Work out the finished part from the listing and answer in its coordinate system (mm). Face numbers are marked on the shaded views. A direction names the side the tool comes from. Coordinates: 2 decimals unless noted, no trailing zeros. Order: outer loops, then holes, each group sorted by start corner. A loop starts at its lowest first (then second) coordinate and runs counter-clockwise, first axis right, second up. Notation, with made-up numbers: (40, -37.5) - (90, -37.5) arc R22 cw to (90, -0.5) - close; hole circle Ø2 at (62.25, 45). An arc over 180 degrees is marked (long way). Answer as a JSON object with one key per item and string values. Group by question number.
1) Section D-D (x = -2.5) is taken. Give the vertices of the cut face in (y, z), plus the area to 3 significant figures.
2) A tool of negligible diameter and unlimited length cuts with its end or side. For the marked faces 5, 6, 7, 8 and 9, from which of +Z, -Z, +X, -X, +Y, -Y can it reach the whole face along a straight path? Write none if from no direction.
3) Each of these flat-tipped pins is pushed along its axis until it touches: P1, Ø1.6, axis at x = 3, y = 0, coming from the -Z side; P2, Ø1, axis at x = -4.5, y = 2, coming from the -Z side; P3, Ø0.9, axis at y = 1, z = 13, coming from the +X side. Where does it stop, or does it pass through?
4) Section B-B (y = -3) is taken. Give the vertices of the cut face in (x, z).
5) The mould has two halves that part along X. Classify the marked faces 1, 2, 3 and 4: released by +X, released by -X, zero draft, split by the parting line, or undercut.
6) Find the intervals of material crossed by line 1 along Y through (x, z) = (8, 11.65); line 2 along Y through (x, z) = (0, 14.5); line 3 along X through (y, z) = (2, 1), in increasing order.
7) Section A-A (x = 8) is taken. Give the vertices of the cut face in (y, z), plus the area to 3 significant figures.
8) Section C-C (z = 9.5) is taken. Give the vertices of the cut face in (x, y), plus the area to 3 significant figures.
from build123d import *

# Parameters (mm, degrees)
PAD_DEPTH       = 15
SKETCH001_W     = 18
SKETCH001_H     = 8
POCKET_DEPTH    = 14
SKETCH002_R     = 1
PAD001_DEPTH    = 2
SKETCH003_R     = 0.5
POCKET001_DEPTH = 15.001
SKETCH004_W     = 8
SKETCH004_H     = 5
SKETCH004_R     = 1.25
PAD002_DEPTH    = 4
SKETCH005_W     = 3.5
SKETCH005_H     = 3
POCKET002_DEPTH = 2.5
POCKET003_DEPTH = 7.501
SKETCH007_W     = 3.5
SKETCH007_H     = 8
PAD003_DEPTH    = 3
SKETCH008_W     = 3
SKETCH008_H     = 3
POCKET004_DEPTH = 2.5
SKETCH010_R     = 0.5
POCKET005_DEPTH = 12.501
SKETCH011_R     = 0.5
POCKET006_DEPTH = 15.001
SKETCH012_W     = 1.058742
SKETCH012_H     = 1
SKETCH012_W_2   = 1.116308
POCKET007_DEPTH = 1


with BuildPart() as part:
    # Sketch → Pad (new body)
    with BuildSketch(Plane.XY):
        with BuildLine():
            Line((-10, 5), (10, 5))
            Line((10, 5), (10, 1.5))
            ThreePointArc((10, -1.5), (11.5, 0), (10, 1.5))
            Line((10, -1.5), (10, -5))
            Line((10, -5), (-10, -5))
            Line((-10, -5), (-10, -1.5))
            ThreePointArc((-10, 1.5), (-11.5, 0), (-10, -1.5))
            Line((-10, 1.5), (-10, 5))
        make_face()
    extrude(amount=PAD_DEPTH)

    # Sketch001 (on Face9 of Pad) → Pocket (cut)
    with BuildSketch(Plane(origin=(0, 0, 0), x_dir=(1, 0, 0), z_dir=(0, 0, -1))):
        Rectangle(SKETCH001_W, SKETCH001_H)
    extrude(amount=-POCKET_DEPTH, mode=Mode.SUBTRACT)

    # Sketch002 (on Face15 of Pocket) → Pad001 (join)
    with BuildSketch(Plane(origin=(0, 0, 14), x_dir=(1, 0, 0), z_dir=(0, 0, -1))):
        with Locations((-2.5, 0)):
            Circle(SKETCH002_R)
        with Locations((2.5, 0)):
            Circle(SKETCH002_R)
    extrude(amount=PAD001_DEPTH)

    # Sketch003 (on Face5 of Pad001) → Pocket001 (cut, through all)
    with BuildSketch(Plane.XY.offset(15)):
        Circle(SKETCH003_R)
    extrude(amount=-POCKET001_DEPTH, mode=Mode.SUBTRACT)

    # Sketch004 (on Face5 of Pocket001) → Pad002 (join)
    with BuildSketch(Plane.XY.offset(15)):
        Rectangle(SKETCH004_W, SKETCH004_H)
        Circle(SKETCH004_R, mode=Mode.SUBTRACT)
    extrude(amount=PAD002_DEPTH)

    # Sketch005 (on Face20 of Pad002) → Pocket002 (cut)
    with BuildSketch(Plane.XY.offset(19)):
        Rectangle(SKETCH005_W, SKETCH005_H)
    extrude(amount=-POCKET002_DEPTH, mode=Mode.SUBTRACT)

    # Sketch006 (on Face16 of Pocket002) → Pocket003 (cut, through all)
    with BuildSketch(Plane.XZ.offset(2.5)):
        with BuildLine():
            ThreePointArc((0.15, 19.022961), (0, 19.172961), (-0.15, 19.022961))
            Line((-0.15, 19.022961), (-0.15, 16.673611))
            ThreePointArc((-0.15, 16.673611), (0, 16.523611), (0.15, 16.673611))
            Line((0.15, 16.673611), (0.15, 19.022961))
        make_face()
    extrude(amount=-POCKET003_DEPTH, mode=Mode.SUBTRACT)

    # Sketch007 (on Face19 of Pocket003) → Pad003 (join)
    with BuildSketch(Plane(origin=(0, 0, 14), x_dir=(1, 0, 0), z_dir=(0, 0, -1))):
        with Locations((7.25, 0)):
            Rectangle(SKETCH007_W, SKETCH007_H)
        with Locations((-7.25, 0)):
            Rectangle(SKETCH007_W, SKETCH007_H)
    extrude(amount=PAD003_DEPTH)

    # Sketch008 (on Face5 of Pad003) → Pocket004 (cut)
    with BuildSketch(Plane.XY.offset(15)):
        with Locations((8.5, -3.5)):
            Rectangle(SKETCH008_W, SKETCH008_H)
        with Locations((8.5, 3.5)):
            Rectangle(SKETCH008_W, SKETCH008_H)
        with Locations((-8.5, -3.5)):
            Rectangle(SKETCH008_W, SKETCH008_H)
        with Locations((-8.5, 3.5)):
            Rectangle(SKETCH008_W, SKETCH008_H)
    extrude(amount=-POCKET004_DEPTH, mode=Mode.SUBTRACT)

    # Sketch010 → Pocket005 (cut, through all)
    with BuildSketch(Plane.XY.offset(12.5)):
        with Locations((8, -3)):
            Circle(SKETCH010_R)
        with Locations((8, 3)):
            Circle(SKETCH010_R)
        with Locations((-8, 3)):
            Circle(SKETCH010_R)
        with Locations((-8, -3)):
            Circle(SKETCH010_R)
    extrude(amount=-POCKET005_DEPTH, mode=Mode.SUBTRACT)

    # Sketch011 (on Face6 of Pocket005) → Pocket006 (cut, through all)
    with BuildSketch(Plane.XY.offset(15)):
        with Locations((-10, 0)):
            Circle(SKETCH011_R)
        with Locations((10, 0)):
            Circle(SKETCH011_R)
    extrude(amount=-POCKET006_DEPTH, mode=Mode.SUBTRACT)

    # Sketch012 (on Face2 of Pocket006) → Pocket007 (cut)
    with BuildSketch(Plane(origin=(0, 0, 0), x_dir=(1, 0, 0), z_dir=(0, 0, -1))):
        with Locations((-9.46722, -1.2e-05)):
            Rectangle(SKETCH012_W, SKETCH012_H)
        with Locations((9.416079, -0.000664)):
            Rectangle(SKETCH012_W_2, SKETCH012_H)
    extrude(amount=-POCKET007_DEPTH, mode=Mode.SUBTRACT)


solid = part.part
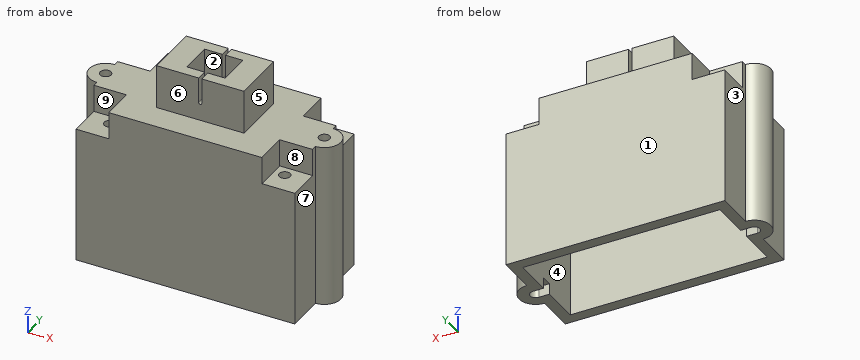
Report:
{
 "1": {"outline": "(-5, 0) - (-4, 0) - (-4, 14) - (-1, 14) - (-1, 12) - (1, 12) - (1, 14) - (4, 14) - (4, 0) - (5, 0) - (5, 15) - (2.5, 15) - (2.5, 19) - (-2.5, 19) - (-2.5, 15) - (-5, 15) - close", "area": "62.0 mm²"},
 "2": {"face 5": "+Z, +X, +Y, -Y", "face 6": "+Z, +X, -X, -Y", "face 7": "+Z, -Z, +X, -Y", "face 8": "+Z, +X, -Y", "face 9": "+Z, -X, -Y"},
 "3": {"P1": "stops at z = 12", "P2": "stops at z = 14", "P3": "stops at x = 11.4"},
 "4": {"outline": "(-10, 0) - (-9, 0) - (-9, 11) - (-8.5, 11) - (-8.5, 12.5) - (-10, 12.5) - close; (-7.5, 11) - (-5.5, 11) - (-5.5, 14) - (5.5, 14) - (5.5, 11) - (7.5, 11) - (7.5, 12.5) - (7, 12.5) - (7, 15) - (-7, 15) - (-7, 12.5) - (-7.5, 12.5) - close; (8.5, 11) - (9, 11) - (9, 0) - (10, 0) - (10, 12.5) - (8.5, 12.5) - close"},
 "5": {"face 1": "zero draft", "face 2": "undercut", "face 3": "released by -X", "face 4": "undercut"},
 "6": {"line 1": "y = -5 to -3.5, -2.5 to 2.5, 3.5 to 5", "line 2": "y = -5 to -0.5, 0.5 to 5", "line 3": "x = -10 to -9, 9 to 10"},
 "7": {"outline": "(-5, 0) - (-4, 0) - (-4, 11) - (-3.5, 11) - (-3.5, 12.5) - (-5, 12.5) - close; (-2.5, 11) - (2.5, 11) - (2.5, 12.5) - (2, 12.5) - (2, 15) - (-2, 15) - (-2, 12.5) - (-2.5, 12.5) - close; (3.5, 11) - (4, 11) - (4, 0) - (5, 0) - (5, 12.5) - (3.5, 12.5) - close", "area": "44.0 mm²"},
 "8": {"outline": "(-10, -5) - (10, -5) - (10, -1.5) arc R1.5 ccw to (10, 1.5) - (10, 5) - (-10, 5) - (-10, 1.5) arc R1.5 ccw to (-10, -1.5) - close; hole circle Ø1 at (-10, 0); hole (-9, -4) - (9, -4) - (9, 4) - (-9, 4) - close; hole circle Ø1 at (10, 0)", "area": "61.5 mm²"}
}
